```python
from build123d import *

# Parameters (mm, degrees)
BASPROSKE_W        = 5
BASPROSKE_H        = 19
TOOTHCUT_DEPTH     = 28.331300737
TEETHCUTS_COUNT    = 17
TEETHCUTS_ANGLE    = 338.823529412
BORSKE_R           = 1.375
BORE_DEPTH         = 50.0000508
SKETCH2_R          = 3.5
CUT_EXTRUDE2_DEPTH = 4
SKETCH1_W          = 15
SKETCH1_H          = 15
CUT_EXTRUDE1_DEPTH = 3


with BuildPart() as part:
    # BasProSke → Base-Revolve (revolve)
    with BuildSketch(Plane(origin=(0, 0, 0), x_dir=(1, 0, 0), z_dir=(0, 1, 0)), mode=Mode.PRIVATE) as base_revolve_sk:
        with Locations((2.5, 9.5)):
            Rectangle(BASPROSKE_W, BASPROSKE_H)
    revolve(base_revolve_sk.sketch.rotate(Axis((-10, 0, 0), (1, 0, 0)), 180), axis=Axis((-10, 0, 0), (1, 0, 0)))

    # TooCutSke → ToothCut (cut, through all)
    with BuildSketch(Plane(origin=(0, 0, 0), x_dir=(0, 0, -1), z_dir=(1, 0, 0))):
        with BuildLine():
            ThreePointArc((1.020352389, 14.463052306), (0, 14.499), (-1.020352389, 14.463052306))
            ThreePointArc((-1.020352389, 14.463052306), (-1.632621885, 16.804485203), (-3.026143023, 18.783192049))
            ThreePointArc((-3.026143023, 18.783192049), (0, 19.0254), (3.026143023, 18.783192049))
            ThreePointArc((3.026143023, 18.783192049), (1.632621885, 16.804485203), (1.020352389, 14.463052306))
        make_face()
    toothcut = extrude(amount=TOOTHCUT_DEPTH, mode=Mode.SUBTRACT)

    # TeethCuts: ToothCut ×17 about axis
    teethcuts_axis = Axis((-10, 0, 0), (1, 0, 0))
    for i in range(1, TEETHCUTS_COUNT):
        add(toothcut.rotate(teethcuts_axis, i * TEETHCUTS_ANGLE / (TEETHCUTS_COUNT - 1)), mode=Mode.SUBTRACT)

    # BorSke → Bore (cut, symmetric)
    with BuildSketch(Plane(origin=(0, 0, 0), x_dir=(0, 0, -1), z_dir=(1, 0, 0))):
        with Locations(Location((0, 0, 0), (0, 0, 180))):
            Circle(BORSKE_R)
    extrude(amount=BORE_DEPTH, both=True, mode=Mode.SUBTRACT)

    # Sketch2 → Cut-Extrude2 (cut)
    with BuildSketch(Plane(origin=(5, 0, 0), x_dir=(0, 0, -1), z_dir=(1, 0, 0))):
        Circle(SKETCH2_R)
    extrude(amount=-CUT_EXTRUDE2_DEPTH, mode=Mode.SUBTRACT)

    # Sketch1 → Cut-Extrude1 (cut)
    with BuildSketch(Plane(origin=(5, 0, 0), x_dir=(0, 0, -1), z_dir=(1, 0, 0))):
        Rectangle(SKETCH1_W, SKETCH1_H)
    extrude(amount=-CUT_EXTRUDE1_DEPTH, mode=Mode.SUBTRACT)


solid = part.part
```
Verification items for the finished model (mm, model axes). A direction names the side the tool comes from. Coordinates: 2 decimals unless noted, no trailing zeros. Loops run counter-clockwise (first coordinate to the right, second up) from the corner with the lowest first, then second, coordinate; pieces in that order, holes last. Notation, with made-up numbers: (58.25, -40) -> (73.25, -40) arc R37 ccw to (73.25, -1) -> close; hole circle Ø5 at (47.25, 3). An arc over 180 degrees is marked (long way). Put each result on its own line as item: value.
1. Gauge pin test, flat ends, axial feed: P1, Ø1.5, axis at x = 3, z = -2.5, coming from the -Y side; P2, Ø1.6, axis at y = 0, z = 0, coming from the +X side; P3, Ø3, axis at x = 2.5, y = -4, coming from the -Z side; P4, Ø5.5, axis at y = 1, z = -1, coming from the +X side. Record the tip position at first contact, or that the pin passes through.
Result set:
P1: stops at y = -14.39
P2: passes through
P3: stops at z = -18.36
P4: stops at x = 2
2. Section check B-B, the plane z = 16. Record the boundary of the cut face in (x, y).
Result set:
outline: (0, -8.97) -> (5, -8.97) -> (5, -6.43) -> (0, -6.43) -> close; (0, -3.1) -> (5, -3.1) -> (5, 0.17) -> (0, 0.17) -> close; (0, 2.87) -> (5, 2.87) -> (5, 6.03) -> (0, 6.03) -> close
3. Thickness scan on line 1 (Y direction, x = 1.3, z = 0); line 2 (Z direction, x = 4.55, y = 0.5); line 3 (Y direction, x = 1.35, z = 15.5). Record the ranges inside material, lowest first.
Result set:
line 1: y = -19 to -3.5, 3.5 to 14.5
line 2: z = -14.49 to -7.5, 7.5 to 14.49
line 3: y = -8.97 to -5.99, -3.11 to 0.26, 2.67 to 6.02
4. Mould release check, pull along Z, two halves, no side actions. Record for faces 6 (the face through (2.54, -17.72, -6.86)), 7 (the face through (2.54, 18.68, 3.48)), 8 (the face through (2.465, 11.326, -12.544)): pulls with the +Z half, pulls with the -Z half, needs draft (parallel to the pull), parting line crosses it, or undercut.
Result set:
face 6: pulls with the -Z half
face 7: pulls with the +Z half
face 8: undercut
5. Tool access check on faces 1 (the face through (2.465, -15.098, 7.452)), 2 (the face through (2.46, -16.23, 4.7)), 3 (the face through (2.46, 11.3, 12.48)), 4 (the face through (2.535, -8.463, 17.011)), 5 (the face through (2.465, -11.386, 12.403)). Record the directions out of +Z, -Z, +X, -X, +Y, -Y that give a thin tool (end or side, any length) a straight path to the whole face; none if there is none.
Result set:
face 1: +X, -X
face 2: +X, -X, -Y
face 3: +X, -X, +Y
face 4: +Z, +X, -X, -Y
face 5: +Z, +X, -X
6. Section check C-C, the plane y = -4.5. Record the boundary of the cut face in (x, z).
Result set:
outline: (0, -13.78) -> (5, -13.78) -> (5, -7.5) -> (2, -7.5) -> (2, 7.5) -> (5, 7.5) -> (5, 13.78) -> (0, 13.78) -> close
7. Section check A-A, the plane z = 0. Record the boundary of the cut face in (x, y) (3 decimals), then the cut area to 3 significant figures.
Result set:
outline: (0, -19) -> (5, -19) -> (5, -7.5) -> (2, -7.5) -> (2, -3.5) -> (1, -3.5) -> (1, -1.375) -> (0, -1.375) -> close; (0, 1.375) -> (1, 1.375) -> (1, 3.5) -> (2, 3.5) -> (2, 7.5) -> (5, 7.5) -> (5, 14.499) -> (0, 14.499) -> close
area: 113 mm^2
